The model under review builds one solid part; all positions refer to its coordinate system, in mm. Face numbers are marked on the shaded views. A direction names the side the tool comes from. Coordinates: 2 decimals unless noted, no trailing zeros. Write each loop counter-clockwise with the first axis right and the second up, starting at its lowest first coordinate (ties: lowest second). Pieces come first, ordered by that corner, then holes. Notation, with made-up numbers: M -9.5,-24.75 L 29.5,-24.75 A17 ccw 29.5,2.25 Z; hole C -26.5,33.5 d10. An arc over 180 degrees is marked long. Answer as a JSON object with one key per item and string values.
Autodesk Inventor part; units mm, degrees
ref_plane "YZ Plane" through (0, 0, 0) normal (1, 0, 0) x (0, 1, 0)
ref_plane "XZ Plane" through (0, 0, 0) normal (0, 1, 0) x (-1, 0, 0)
ref_plane "XY Plane" through (0, 0, 0) normal (0, 0, 1) x (1, 0, 0)
sketch "Boceto1" plane through (0, 0, 0) normal (0, 1, 0) x (-1, 0, 0)
  line L0 (2.3676, 25.5961) -> (2.3676, 5.5961)
  line L1 (-23.6324, 5.5961) -> (-23.6324, 25.5961)
  line L2 (-23.6324, 25.5961) -> (2.3676, 25.5961)
  line L3 (2.3676, 25.5961) -> (2.3676, 5.5961)
  circle A0 centre (-16.1599, -0.9039) radius 2.5
  circle A1 centre (-4.9324, 15.5961) radius 2.5
  circle A2 centre (-10.6324, -50.9039) radius 2.5
  line L4 (2.3676, 5.5961) -> (-7.173, -56.436)
  line L5 (-14.0917, -56.436) -> (-23.6324, 5.5961)
  arc A3 (-14.0917, -56.436) -> (-7.173, -56.436) centre (-10.6324, -55.9039) ccw
  circle A4 centre (-10.6324, -30.9039) radius 2.5
  point P0 (0, 0)
  dimension "d2" = 20
  dimension "d16" = 26
  dimension "d17" = 5
  dimension "d18" = 5
  dimension "d19" = 5
  dimension "d20" = 10
  dimension "d21" = 7.3
  dimension "d22" = 26.5
  dimension "d26" = 5
  dimension "d30" = 5
  dimension "d31" = 20
extrude "Extrusión1" add sketch "Boceto1" along normal blind 1.2
sketch "Boceto4" plane through (23.6324, 0, 25.5961) normal (1, 0, 0) x (0, 0, -1)
  circle A0 centre (-2.375, -1.175) radius 2.375
  circle A1 centre (-2.375, -1.175) radius 1.625
  line L0 (0, 0) -> (0, 1.2)
  line L1 (0, 1.2) -> (20, 1.2)
  line L2 (20, 1.2) -> (0, 1.2)
  line L3 (0, 1.2) -> (-2.375, 1.2)
  line L4 (20, 0) -> (0, 0)
  line L5 (0, 0) -> (0, -1.175)
  point P0 (25.5961, 0)
  point P1 (20, 2)
  dimension "d12" = 4.75
  dimension "d13" = 3.25
extrude "Extrusión3" add sketch "Boceto4" against normal blind 26
chamfer "Chaflán1" distance 0.25 angle 45 4 edges at (7.4324, 0, 15.5961) (18.6599, 0, -0.9039) (13.1324, 0, -50.9039) (13.1324, 0, -30.9039)
properties part number "Ala 2 Bisagra tipo T"
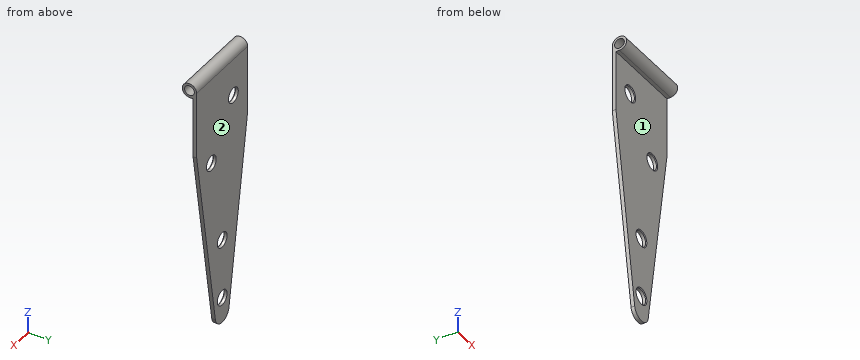
(1) For the marked faces 1 and 2, list the 3-axis set-ups (+Z, -Z, +X, -X, +Y, -Y) from which the entire face can be reached by the end or side of a thin tool; tool diameter is ignored.
Results list:
{"face 1": "-Z, +X, -X, -Y", "face 2": "+Z, -Z, +X, -X, +Y"}
(2) Add section A-A on x = 11.5. Count the separate pieces of the cut face and the enclosed holes in it, and give its area (3 significant figures).
Results list:
{"separate pieces": "3", "enclosed holes": "1", "area": "101 mm²"}
(3) Wall thickness on line 1 along Z through (x, y) = (6.75, -1.1); line 2 along Y through (x, z) = (9.25, -35.5): over which ranges is each line inside the solid? List them lowest first. Write a range as from..to.
Results list:
{"line 1": "25.6..26.35, 29.59..30.34", "line 2": "0..1.2"}
(4) Add section D-D on x = 0. Give the boundary of the cut face in (y, z) (3 decimals).
Results list:
{"outline": "M -1.175,25.596 L 0,25.596 L 0,-9.798 L 1.2,-9.798 L 1.2,27.971 A2.375 ccw long Z; hole C -1.175,27.971 d3.25"}
(5) Add section C-C on z = 9.5. Give the boundary of the cut face in (x, y), and give its area (3 significant figures).
Results list:
{"outline": "M -2.37,0 L 23.63,0 L 23.63,1.2 L -2.37,1.2 Z", "area": "31.2 mm²"}
(6) Add section B-B on x = 20.75. Give the boundary of the cut face in (y, z) (3 decimals), and give its area (3 significant figures).
Results list:
{"outline": "M -1.175,25.596 L 0,25.596 L 0,-13.145 L 1.2,-13.145 L 1.2,27.971 A2.375 ccw long Z; hole C -1.175,27.971 d3.25", "area": "57.1 mm²"}
(7) For pin 1 Ø6.5 at (x, z) = (10.63, -30.9) entering from -Y; pin 2 Ø1.5 at (y, z) = (-0.5, -40.5) entering from -X; pin 3 Ø1 at (x, y) = (12, -2) entering from -Z, all flat-tipped, find the tip position at first contact; note any pin that passes through.
Results list:
{"pin 1": "y = 0", "pin 2": "x = 4.64", "pin 3": "z = 25.62"}
